Read the model definition and answer for the solid it produces. Units are mm, in the model's axes. A direction names the side the tool comes from. Coordinates: 2 decimals unless noted, no trailing zeros. Write each loop counter-clockwise with the first axis right and the second up, starting at its lowest first coordinate (ties: lowest second). Pieces come first, ordered by that corner, then holes.
Item 1: A tool of negligible diameter and unlimited length cuts with its end or side. For faces 1 (the face through (-26.428, -7.509, 23.846)), 2 (the face through (-39, -84, -56)), 3 (the face through (23.068, 104.456, -23.196)), 4 (the face through (-1, -15.5, 0)), 5 (the face through (11, 20, -20)), from which of +Z, -Z, +X, -X, +Y, -Y can it reach the whole face along a straight path? Write none if from no direction.
Item 2: Section B-B (z = -6) is taken. State how many separate pieces and enclosed holes the cut face has, then the cut area to 3 significant figures.
Item 3: Straight lines are drawn through the part: probe 1 along Z at (x, y) = (14, 0); probe 2 along Z at (x, y) = (34, -7); probe 3 along X at (y, z) = (99, 51). For each, find the intervals that lie inside material, in ascending order.
Item 4: Determine the mould class of faces 6 (the face through (39, -11.5, 5.9)), 7 (the face through (-0.154, 80.483, 0.791)), 8 (the face through (11.52, -5.5, -124.88)) for opening direction Y: released by +Y, released by -Y, zero draft, split by the parting line, or undercut.
Item 5: Section A-A (x = 29.5) is taken. Give the vertices of the cut face in (y, z), then the cut area to 3 significant figures.
Item 6: Each of these flat-tipped pins is pushed along its axis until it touches: P1, Ø8, axis at x = -23.5, z = -1.5, coming from the +Y side; P2, Ø3, axis at x = 24, y = 38.5, coming from the -Z side; P3, Ø4, axis at x = 27.5, y = 48, coming from the -Z side. Where does it stop, or does it pass through?
from build123d import *

# Parameters (mm, degrees)
F2_R     = 18
F3_DEPTH = 50.001
F5_DEPTH = 78.001
F6_R     = 2.5


with BuildPart() as f1:
    # F0 (on Front) → F1 (revolve)
    with BuildSketch(Plane.XZ):
        Polygon((-11, 25), (-39, 25), (-39, 12.5), (39, 12.5), (39, 25), (11, 25), (11, 100), (39, 100), (39, 125), (34, 125), (25.602928, 107), (20.602928, 107), (14.051464, 125), (9.051464, 125), (2.5, 107), (-2.5, 107), (-9.051464, 125), (-14.051464, 125), (-20.602928, 107), (-25.602928, 107), (-34, 125), (-39, 125), (-39, 100), (-11, 100), align=None)
    revolve(axis=Axis((0, 0, 0), (1, 0, 0)))

    # F2 (on face) → F3 (cut, through all)
    with BuildSketch(Plane(origin=(-11, 0, 0), x_dir=(0, -1, 0), z_dir=(-1, 0, 0))):
        with Locations((-62.5, 0)):
            Circle(F2_R)
        with Locations((0, -62.5)):
            Circle(F2_R)
        with Locations((62.5, 0)):
            Circle(F2_R)
        with Locations((0, 62.5)):
            Circle(F2_R)
    extrude(amount=-F3_DEPTH, mode=Mode.SUBTRACT)

    # F4 (on face) → F5 (cut, through all)
    with BuildSketch(Plane(origin=(-39, 0, 0), x_dir=(0, -1, 0), z_dir=(-1, 0, 0))):
        with BuildLine():
            Line((15.5, 3), (12.134661, 3))
            ThreePointArc((12.134661, 3), (12.408329, 1.511082), (12.5, 0))
            ThreePointArc((12.5, 0), (12.408329, -1.511082), (12.134661, -3))
            Line((12.134661, -3), (15.5, -3))
            Line((15.5, -3), (15.5, 3))
        make_face()
    extrude(amount=-F5_DEPTH, mode=Mode.SUBTRACT)

    # F6
    f6_edges = [f1.edges().sort_by_distance(p)[0] for p in [
        (-11, 0, -100),
        (-11, 0, -25),
        (11, 0, -25),
        (11, 0, -100),
    ]]
    fillet(f6_edges, radius=F6_R)


solid = f1.part
Established:
1. face 1: -X
1. face 2: +Z, -Z, -X, +Y, -Y
1. face 3: none
1. face 4: +X, -X
1. face 5: +X
2. separate pieces: 4
2. enclosed holes: 0
2. area: 6,510 mm2
3. probe 1: z = -125 to -100, -25 to -12.5, 12.5 to 25, 100 to 125
3. probe 2: z = -124.8 to -99.75, -24 to -10.36, 10.36 to 24, 99.75 to 124.8
3. probe 3: x = -39 to -27.64, -19.01 to -4.09, 4.09 to 19.01, 27.64 to 39
4. face 6: zero draft
4. face 7: undercut
4. face 8: split by the parting line
5. outline: circle Ø230.71 at (0, 0); circle Ø50 at (0, 0); hole circle Ø200 at (0, 0); hole (-15.5, -3) - (-12.13, -3) arc R12.5 ccw (long way) to (-12.13, 3) - (-15.5, 3) - close
5. area: 11,800 mm2
6. P1: stops at y = 111.06
6. P2: stops at z = -100.4
6. P3: stops at z = -104.98
